from build123d import *

# Parameters (mm, degrees)
SKETCH2_R           = 2
SKETCH2_R_2         = 1.999999991
BOSS_EXTRUDE1_DEPTH = 5.588
SKETCH7_R           = 2.032
CUT_EXTRUDE1_DEPTH  = 5.588
CUT_EXTRUDE2_DEPTH  = 226.492641696


with BuildPart() as part:
    # Sketch2 → Boss-Extrude1 (new body)
    with BuildSketch(Plane(origin=(0, 0, 0), x_dir=(1, 0, 0), z_dir=(0, 1, 0))):
        with BuildLine():
            ThreePointArc((17.295902343, -29.323452593), (16.73639375, -27.733089808), (15.304363929, -26.843373987))
            Line((15.304363929, -26.843373987), (13.284423018, -26.396670406))
            ThreePointArc((13.284423018, -26.396670406), (11.420627025, -25.189010374), (10.804170553, -23.055431298))
            Line((10.804170553, -23.055431298), (12.5603, 0))
            ThreePointArc((12.5603, 0), (0.640974044, 12.543934326), (-12.49487995, 1.28027775))
            Line((-12.49487995, 1.28027775), (-16.496770465, -37.776201638))
            ThreePointArc((-16.496770465, -37.776201638), (-16.50669046, -37.90548449), (-16.51, -38.035105126))
            Line((-16.51, -38.035105126), (-16.51, -220.313887427))
            ThreePointArc((-16.51, -220.313887427), (-12.970187584, -224.665744552), (-7.988667969, -222.086327038))
            Line((-7.988667969, -222.086327038), (16.979901226, -164.662549258))
            ThreePointArc((16.979901226, -164.662549258), (17.216065593, -163.919190378), (17.295902343, -163.143315306))
            Line((17.295902343, -163.143315306), (17.295902343, -29.323452593))
        make_face()
        with Locations(Location((-11.43, -219.075, 0), (0, 0, 270))):
            Circle(SKETCH2_R, mode=Mode.SUBTRACT)
        with Locations(Location((-11.43, -212.725, 0), (0, 0, 270))):
            Circle(SKETCH2_R, mode=Mode.SUBTRACT)
        with Locations(Location((-11.43, -206.375, 0), (0, 0, 270))):
            Circle(SKETCH2_R, mode=Mode.SUBTRACT)
        with Locations(Location((-11.43, -200.025, 0), (0, 0, 270))):
            Circle(SKETCH2_R, mode=Mode.SUBTRACT)
        with BuildLine():
            ThreePointArc((7.135902343, -161.395796446), (8.023611961, -164.633987883), (10.438542905, -166.966801782))
            Line((10.438542905, -166.966801782), (-0.894016375, -193.029903785))
            ThreePointArc((-0.894016375, -193.029903785), (-2.665854515, -194.495144898), (-4.89449504, -193.929898651))
            Line((-4.89449504, -193.929898651), (-11.831146076, -187.869646091))
            ThreePointArc((-11.831146076, -187.869646091), (-12.472607947, -187.007278248), (-12.7, -185.95682859))
            Line((-12.7, -185.95682859), (-12.7, -146.861981888))
            ThreePointArc((-12.7, -146.861981888), (-11.955224829, -145.705677915), (-10.594426962, -145.905573138))
            Line((-10.594426962, -145.905573138), (7.135902343, -161.395796446))
        make_face(mode=Mode.SUBTRACT)
        with BuildLine():
            ThreePointArc((12.215902343, -151.955842791), (10.785297541, -152.261664921), (9.418398214, -152.782955151))
            Line((9.418398214, -152.782955151), (-10.962292152, -134.977225798))
            ThreePointArc((-10.962292152, -134.977225798), (-12.245215894, -133.252490112), (-12.7, -131.151590796))
            Line((-12.7, -131.151590796), (-12.7, -90.4875))
            ThreePointArc((-12.7, -90.4875), (-11.765673597, -90.432318214), (-10.844338135, -90.267540106))
            Line((-10.844338135, -90.267540106), (11.513275375, -128.23323342))
            ThreePointArc((11.513275375, -128.23323342), (12.037098881, -129.475107855), (12.215902343, -130.811024207))
            Line((12.215902343, -130.811024207), (12.215902343, -151.955842791))
        make_face(mode=Mode.SUBTRACT)
        with Locations(Location((13.485902343, -161.395796446, 0), (0, 0, 270))):
            Circle(SKETCH2_R, mode=Mode.SUBTRACT)
        with BuildLine():
            Line((-10.16, -41.91), (2.838491406, -41.91))
            ThreePointArc((2.838491406, -41.91), (3.914572403, -42.505500417), (3.981509018, -43.733543799))
            Line((3.981509018, -43.733543799), (-11.055993219, -74.784618621))
            ThreePointArc((-11.055993219, -74.784618621), (-11.873503915, -74.655646925), (-12.7, -74.6125))
            Line((-12.7, -74.6125), (-12.7, -44.45))
            ThreePointArc((-12.7, -44.45), (-11.956051224, -42.653948776), (-10.16, -41.91))
        make_face(mode=Mode.SUBTRACT)
        with BuildLine():
            ThreePointArc((-9.886442157, -38.1), (-11.771808813, -37.262055396), (-12.413212622, -35.301096512))
            Line((-12.413212622, -35.301096512), (-9.81475239, -9.941405108))
            ThreePointArc((-9.81475239, -9.941405108), (-3.431386466, -13.542026692), (3.896359547, -13.415635739))
            Line((3.896359547, -13.415635739), (2.194931831, -35.752912681))
            ThreePointArc((2.194931831, -35.752912681), (1.388767881, -37.42300808), (-0.337731726, -38.1))
            Line((-0.337731726, -38.1), (-9.886442157, -38.1))
        make_face(mode=Mode.SUBTRACT)
        with BuildLine():
            ThreePointArc((3.111707299, -3.622128204), (-4.505881672, 1.581001391), (4.69270869, 0.883753468))
            Line((4.69270869, 0.883753468), (3.111707299, -3.622128204))
        make_face(mode=Mode.SUBTRACT)
        with BuildLine():
            ThreePointArc((-8.804706991, -86.222769023), (-8.262040897, -82.55), (-8.804706991, -78.877230977))
            Line((-8.804706991, -78.877230977), (8.75092063, -42.626456201))
            ThreePointArc((8.75092063, -42.626456201), (9.219438659, -42.103919003), (9.893938242, -41.91))
            Line((9.893938242, -41.91), (10.945902343, -41.91))
            ThreePointArc((10.945902343, -41.91), (11.843927955, -42.281974388), (12.215902343, -43.18))
            Line((12.215902343, -43.18), (12.215902343, -62.618124667))
            ThreePointArc((12.215902343, -62.618124667), (6.906756389, -72.428110561), (13.516748759, -81.413145613))
            Line((13.516748759, -81.413145613), (13.516748759, -119.431411199))
            ThreePointArc((13.516748759, -119.431411199), (12.599191369, -120.688899116), (11.152950849, -120.113072943))
            Line((11.152950849, -120.113072943), (-8.804706991, -86.222769023))
        make_face(mode=Mode.SUBTRACT)
        with Locations(Location((13.485902343, -38.1, 0), (0, 0, 270))):
            Circle(SKETCH2_R_2, mode=Mode.SUBTRACT)
    extrude(amount=BOSS_EXTRUDE1_DEPTH)

    # Sketch7 → Cut-Extrude1 (cut)
    with BuildSketch(Plane(origin=(0, 5.588, 0), x_dir=(1, 0, 0), z_dir=(0, 1, 0))):
        with Locations(Location((12.215902343, -72.362149281, 0), (0, 0, 270))):
            Circle(SKETCH7_R)
    extrude(amount=-CUT_EXTRUDE1_DEPTH, mode=Mode.SUBTRACT)

    # Sketch8 → Cut-Extrude2 (cut, through all)
    with BuildSketch(Plane(origin=(0, 5.588, 0), x_dir=(1, 0, 0), z_dir=(0, 1, 0))):
        Polygon((1.820727883, 5.189106375), (-3.583534002, 4.171349788), (-5.404261886, -1.017756587), (-1.820727883, -5.189106375), (3.583534002, -4.171349788), (5.404261886, 1.017756587), align=None)
    extrude(amount=-CUT_EXTRUDE2_DEPTH, mode=Mode.SUBTRACT)


solid = part.part
Input: part model. Units: mm. Frame: model coordinates. A direction names the side the tool comes from. Coordinates: 2 decimals unless noted, no trailing zeros. Order: outer loops, then holes, each group sorted by start corner. A loop starts at its lowest first (then second) coordinate and runs counter-clockwise, first axis right, second up. Notation, with made-up numbers: M -31,-11.5 L -17,-11.5 A11 cw -17,2.5 Z; hole C -5.75,-36.75 d10. An arc over 180 degrees is marked long. Answer as CSV lines item,"result".
1. Access query for faces 4 (the flat face through (11.67, 2.75, 11.69)), 5 (the flat face through (-4, 3, 41.91)), 6 (the flat face through (0, 0, 104)). Directions: +Z, -Z, +X, -X, +Y, -Y. A direction counts if a zero-diameter tool reaches every point of the face in a straight line with its end or side. Return the directions, or none.
Reported:
face 4,"+X, +Y, -Y"
face 5,"+Y, -Y"
face 6,"+Z, -Z, +X, -X, -Y"
2. First-contact query: P1, Ø0.8, axis at x = 10.5, y = 3.5, coming from the +Z side; P2, Ø2, axis at x = -10, y = 3.5, coming from the -Z side; P3, Ø3, axis at x = -5, y = 3, coming from the +Z side. Flat tips, straight axial feed; report the tip coordinate or a pass-through.
Reported:
P1,"z = 180.49"
P2,"z = -8.76"
P3,"z = 218.66"
3. Material intervals for line 1 (X direction, y = 4.8, z = 83); line 2 (X direction, y = 4.4, z = 69.5); line 3 (X direction, y = 2.75, z = 119), sorted ascending. Write a range as from..to.
Reported:
line 1,"-16.51..-8.27, 13.52..17.3"
line 2,"-16.51..-12.7, -8.5..-4.26, 7.12..17.3"
line 3,"-16.51..-12.7, 6.08..10.5, 13.52..17.3"
4. Section A-A (z = 103). Return the cut outline in (x, y).
Reported:
outline,"M -16.51,0 L -12.7,0 L -12.7,5.59 L -16.51,5.59 Z; M -3.35,0 L 1.08,0 L 1.08,5.59 L -3.35,5.59 Z; M 13.52,0 L 17.3,0 L 17.3,5.59 L 13.52,5.59 Z"
5. Section B-B (y = 3.7). State how many separate pieces and enclosed holes the cut face has, then the cut area to 3 significant figures.
Reported:
separate pieces,"1"
enclosed holes,"13"
area,"3,400 mm2"
6. Pull-direction query (Z, two-part tool) for faces 1 (the cylindrical face through (0.908, 2.755, -12.527)), 2 (the flat face through (17.296, 3, 97)), 3 (the flat face through (12.216, 3, 53)); classes: released by +Z, released by -Z, zero draft, split by the parting line, or undercut.
Reported:
face 1,"released by -Z"
face 2,"zero draft"
face 3,"undercut"
